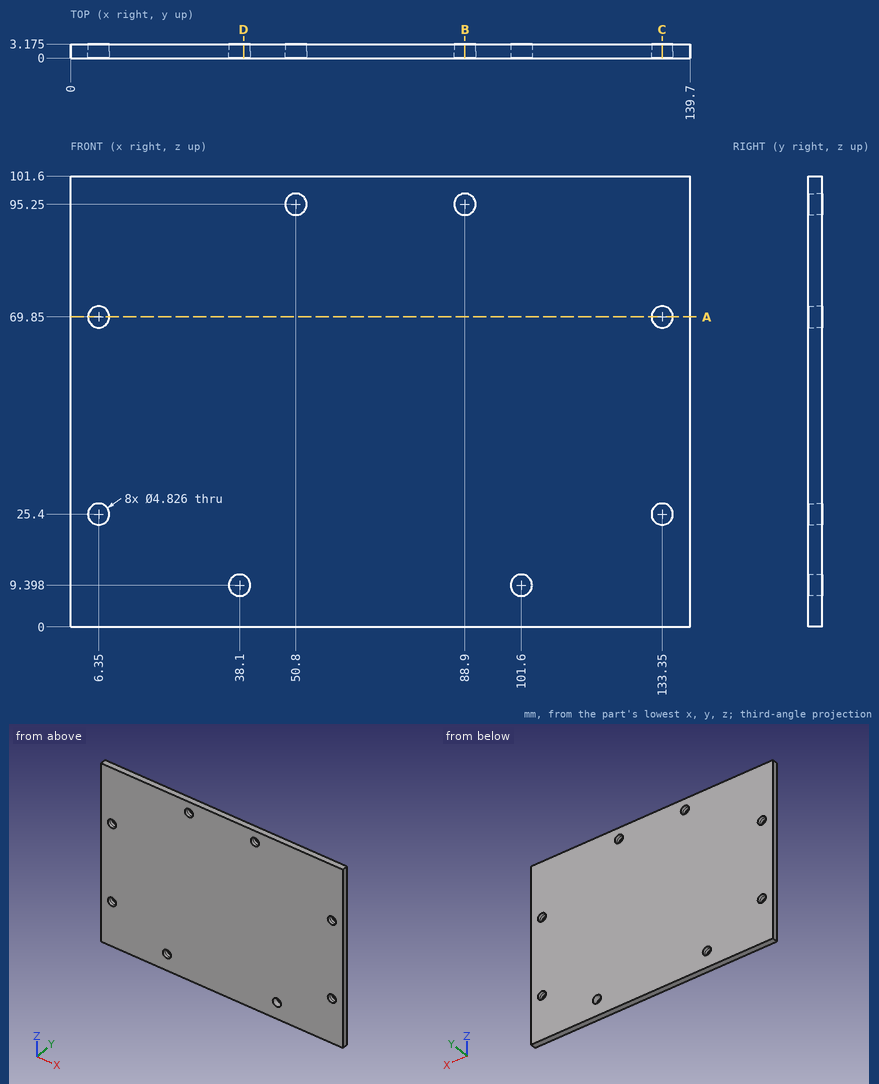
For this review, use the dimensioned drawing (mm, ordinates from the lowest corner) and the shaded views. Coordinates: 2 decimals unless noted, no trailing zeros. Loops run counter-clockwise (first coordinate to the right, second up) from the corner with the lowest first, then second, coordinate; pieces in that order, holes last.
1. Add section A-A, the plane z = 69.85. Give the boundary of the cut face in (x, y) (3 decimals), then the cut area to 3 significant figures.
2. Add section C-C, the plane x = 133.35. Give the boundary of the cut face in (y, z) (3 decimals).
3. Add section D-D, the plane x = 39. Give the boundary of the cut face in (y, z) (3 decimals).
4. For line 1 (Z direction, x = 6.35, y = 2.45); line 2 (X direction, y = 0.45, z = 25.4); line 3 (Z direction, x = 88.9, y = 0.45), list the stretches that pass through material, from the lowest coordinate up.
5. Insertion check: P1, Ø4, axis at x = 6.35, z = 25.4, coming from the +Y side. The pin has a flat end and moves straight along its axis. Give the tip position at first contact, or say it passes through.
6. Add section B-B, the plane x = 88.9. Give the boundary of the cut face in (y, z) (3 decimals), then the cut area to 3 significant figures.
Result:
1. outline: (0, 0) - (3.937, 0) - (3.937, 3.175) - (0, 3.175) - close; (8.763, 0) - (130.937, 0) - (130.937, 3.175) - (8.763, 3.175) - close; (135.763, 0) - (139.7, 0) - (139.7, 3.175) - (135.763, 3.175) - close
1. area: 413 mm2
2. outline: (0, 0) - (3.175, 0) - (3.175, 22.987) - (0, 22.987) - close; (0, 27.813) - (3.175, 27.813) - (3.175, 67.437) - (0, 67.437) - close; (0, 72.263) - (3.175, 72.263) - (3.175, 101.6) - (0, 101.6) - close
3. outline: (0, 0) - (3.175, 0) - (3.175, 7.159) - (0, 7.159) - close; (0, 11.637) - (3.175, 11.637) - (3.175, 101.6) - (0, 101.6) - close
4. line 1: z = 0 to 22.99, 27.81 to 67.44, 72.26 to 101.6
4. line 2: x = 0 to 3.94, 8.76 to 130.94, 135.76 to 139.7
4. line 3: z = 0 to 92.84, 97.66 to 101.6
5. P1: passes through
6. outline: (0, 0) - (3.175, 0) - (3.175, 92.837) - (0, 92.837) - close; (0, 97.663) - (3.175, 97.663) - (3.175, 101.6) - (0, 101.6) - close
6. area: 307 mm2
